Input: part model. Units: mm. Frame: model coordinates. Coordinates: 2 decimals unless noted, no trailing zeros. Order: outer loops, then holes, each group sorted by start corner. A loop starts at its lowest first (then second) coordinate and runs counter-clockwise, first axis right, second up. Notation, with made-up numbers: (39.25, 34) -> (54.25, 34) arc R8 cw to (54.25, 42) -> close; hole circle Ø6 at (-23.75, 67.5). An arc over 180 degrees is marked (long way). Write each question's results on one line, items separated by ' | '.
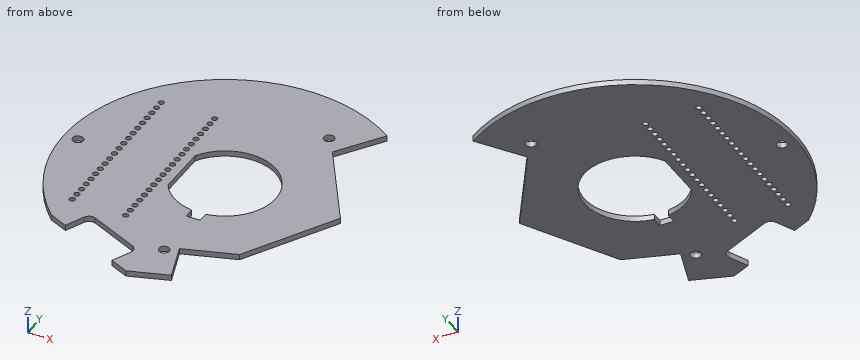
```python
from build123d import *

# Parameters (mm, degrees)
BOSS_EXTRUDE1_DEPTH = 1.6
CUT_EXTRUDE1_DEPTH  = 1.6
SKETCH3_W           = 4
SKETCH3_H           = 3
CUT_EXTRUDE2_DEPTH  = 1.6
SKETCH4_R           = 1.5
CUT_EXTRUDE3_DEPTH  = 5
SKETCH5_R           = 0.8
CUT_EXTRUDE4_DEPTH  = 10
CUT_EXTRUDE5_DEPTH  = 10
CUT_EXTRUDE6_DEPTH  = 5
FILLET1_R           = 2


with BuildPart() as part:
    # Sketch1 → Boss-Extrude1 (new body)
    with BuildSketch(Plane.XY):
        with BuildLine():
            Line((17.486502451, 24.97331362), (26.384516072, 37.680994037))
            ThreePointArc((26.384516072, 37.680994037), (-35.308070708, 29.48457466), (-32.372261705, -32.680830346))
            Line((-32.372261705, -32.680830346), (-4.226479762, -45.805424011))
            ThreePointArc((-4.226479762, -45.805424011), (1.848027324, -45.962863216), (7.890286138, -45.318245604))
            Line((7.890286138, -45.318245604), (3.181347574, -30.825622907))
            Line((3.181347574, -30.825622907), (17.866632614, -26.054084553))
            Line((17.866632614, -26.054084553), (32.908965344, 0))
            Line((32.908965344, 0), (17.486502451, 24.97331362))
        make_face()
    extrude(amount=BOSS_EXTRUDE1_DEPTH)

    # Sketch2 → Cut-Extrude1 (cut)
    with BuildSketch(Plane.XY.offset(1.6)):
        with BuildLine():
            Line((-12.439410298, 7.331960256), (-12.439410298, -7.331960256))
            ThreePointArc((-12.439410298, -7.331960256), (14.439410298, 0), (-12.439410298, 7.331960256))
        make_face()
    extrude(amount=-CUT_EXTRUDE1_DEPTH, mode=Mode.SUBTRACT)

    # Sketch3 → Cut-Extrude2 (cut)
    with BuildSketch(Plane.XY.offset(1.6)):
        with Locations((0, -15.80022971)):
            Rectangle(SKETCH3_W, SKETCH3_H)
    extrude(amount=-CUT_EXTRUDE2_DEPTH, mode=Mode.SUBTRACT)

    # Sketch4 → Cut-Extrude3 (cut)
    with BuildSketch(Plane.XY.offset(1.6)):
        with Locations((-42, 0)):
            Circle(SKETCH4_R)
        with Locations((13.946402637, 29.908156972)):
            Circle(SKETCH4_R)
        with Locations((0, -33)):
            Circle(SKETCH4_R)
    extrude(amount=-CUT_EXTRUDE3_DEPTH, mode=Mode.SUBTRACT)

    # Sketch5 → Cut-Extrude4 (cut)
    with BuildSketch(Plane.XY.offset(1.6)):
        with Locations((-30.919410298, -24.13)):
            Circle(SKETCH5_R)
        with Locations((-15.679410309, -24.13)):
            Circle(SKETCH5_R)
        with Locations((-30.919410298, -21.59)):
            Circle(SKETCH5_R)
        with Locations((-15.679410309, -21.59)):
            Circle(SKETCH5_R)
        with Locations((-30.919410298, -19.05)):
            Circle(SKETCH5_R)
        with Locations((-15.679410309, -19.05)):
            Circle(SKETCH5_R)
        with Locations((-30.919410298, -16.51)):
            Circle(SKETCH5_R)
        with Locations((-15.679410309, -16.51)):
            Circle(SKETCH5_R)
        with Locations((-30.919410298, -13.97)):
            Circle(SKETCH5_R)
        with Locations((-15.679410309, -13.97)):
            Circle(SKETCH5_R)
        with Locations((-30.919410298, -11.43)):
            Circle(SKETCH5_R)
        with Locations((-15.679410309, -11.43)):
            Circle(SKETCH5_R)
        with Locations((-30.919410298, -8.89)):
            Circle(SKETCH5_R)
        with Locations((-15.679410309, -8.89)):
            Circle(SKETCH5_R)
        with Locations((-30.919410298, -6.35)):
            Circle(SKETCH5_R)
        with Locations((-15.679410309, -6.35)):
            Circle(SKETCH5_R)
        with Locations((-30.919410298, -3.81)):
            Circle(SKETCH5_R)
        with Locations((-15.679410309, -3.81)):
            Circle(SKETCH5_R)
        with Locations((-30.919410298, -1.27)):
            Circle(SKETCH5_R)
        with Locations((-15.679410309, -1.27)):
            Circle(SKETCH5_R)
        with Locations((-30.919410298, 1.27)):
            Circle(SKETCH5_R)
        with Locations((-15.679410309, 1.27)):
            Circle(SKETCH5_R)
        with Locations((-30.919410298, 3.81)):
            Circle(SKETCH5_R)
        with Locations((-15.679410309, 3.81)):
            Circle(SKETCH5_R)
        with Locations((-30.919410298, 6.35)):
            Circle(SKETCH5_R)
        with Locations((-15.679410309, 6.35)):
            Circle(SKETCH5_R)
        with Locations((-30.919410298, 8.89)):
            Circle(SKETCH5_R)
        with Locations((-15.679410309, 8.89)):
            Circle(SKETCH5_R)
        with Locations((-30.919410298, 11.43)):
            Circle(SKETCH5_R)
        with Locations((-15.679410309, 11.43)):
            Circle(SKETCH5_R)
        with Locations((-30.919410298, 13.97)):
            Circle(SKETCH5_R)
        with Locations((-15.679410309, 13.97)):
            Circle(SKETCH5_R)
        with Locations((-30.919410298, 16.51)):
            Circle(SKETCH5_R)
        with Locations((-15.679410309, 16.51)):
            Circle(SKETCH5_R)
        with Locations((-30.919410298, 19.05)):
            Circle(SKETCH5_R)
        with Locations((-15.679410309, 19.05)):
            Circle(SKETCH5_R)
        with Locations((-30.919410298, 21.59)):
            Circle(SKETCH5_R)
        with Locations((-15.679410309, 21.59)):
            Circle(SKETCH5_R)
        with Locations((-30.919410298, 24.13)):
            Circle(SKETCH5_R)
        with Locations((-15.679410309, 24.13)):
            Circle(SKETCH5_R)
    extrude(amount=-CUT_EXTRUDE4_DEPTH, mode=Mode.SUBTRACT)

    # Sketch6 → Cut-Extrude5 (cut)
    with BuildSketch(Plane.XY.offset(1.6)):
        Polygon((-4.226479762, -45.805424011), (6.876416094, -42.197874462), (21.084325359, -57.487819449), (-10.029151778, -66.166531288), align=None)
    extrude(amount=-CUT_EXTRUDE5_DEPTH, mode=Mode.SUBTRACT)

    # Sketch7 → Cut-Extrude6 (cut)
    with BuildSketch(Plane.XY.offset(1.6)):
        Polygon((-27.117745501, -35.131051492), (-23.736799407, -27.880589196), (-6.100049872, -36.104740569), (-9.480995966, -43.355202865), align=None)
    extrude(amount=-CUT_EXTRUDE6_DEPTH, mode=Mode.SUBTRACT)

    # Fillet1
    fillet1_edges = [part.edges().sort_by_distance(p)[0] for p in [
        (-23.736799407, -27.880589196, 0.8),
        (-6.100049872, -36.104740569, 0.8),
    ]]
    fillet(fillet1_edges, radius=FILLET1_R)


solid = part.part
```
(1) Cut plane B-B, the plane x = 0. Return loops of the section in (y, z), plus the area to 3 significant figures.
Return value:
outline: (-44.43, 0) -> (-34.5, 0) -> (-34.5, 1.6) -> (-44.43, 1.6) -> close; (-31.5, 0) -> (-17.3, 0) -> (-17.3, 1.6) -> (-31.5, 1.6) -> close; (14.44, 0) -> (46, 0) -> (46, 1.6) -> (14.44, 1.6) -> close | area: 89.1 mm2
(2) Cut plane A-A, the plane x = 25. Return loops of the section in (y, z).
Return value:
outline: (-13.7, 0) -> (12.81, 0) -> (12.81, 1.6) -> (-13.7, 1.6) -> close; (35.7, 0) -> (38.61, 0) -> (38.61, 1.6) -> (35.7, 1.6) -> close
(3) Pin query (flat end, axial travel): P1, Ø1.3, axis at x = -15.68, y = 13.97, coming from the -Z side; P2, Ø2, axis at x = -30.92, y = -1.27, coming from the +Z side; P3, Ø0.8, axis at y = -15, z = 1, coming from the -X side. Return the tip coordinate at first contact, or that it passes through.
Return value:
P1: through | P2: z = 1.6 | P3: x = -43.62
(4) Cut plane C-C, the plane z = 0.9. Count the separate pieces of the cut face and the enclosed holes in it, plus the area to 3 significant figures.
Return value:
separate pieces: 1 | enclosed holes: 44 | area: 4,200 mm2
(5) Line query: line 1 along X through (y, z) = (-32, 0.55); line 2 along Y through (x, z) = (0, 0.45); line 3 along X through (y, z) = (-16.5, 1.5). Output: solid intervals per line, ascending. Write a range as from..to.
Return value:
line 1: -33.05..-25.66, -14.9..-1.12, 1.12..3.56 | line 2: -44.43..-34.5, -31.5..-17.3, 14.44..46 | line 3: -42.94..-31.72, -30.12..-16.48, -14.88..-2, 2..23.38
(6) Cut plane D-D, the plane y = 27. Return loops of the section in (x, z), plus the area to 3 significant figures.
Return value:
outline: (-37.24, 0) -> (18.91, 0) -> (18.91, 1.6) -> (-37.24, 1.6) -> close | area: 89.8 mm2
